from build123d import *

# Parameters (mm, degrees)
F0_R     = 3.3
F1_DEPTH = 5
F2_W     = 33
F2_H     = 6.5
F2_W_2   = 28
F3_DEPTH = 2


# Not quite as in the source:
# - a feature names something its author has since deleted; it is built from what else it names


with BuildPart() as f1:
    # F0 (on Front) → F1 (new body)
    with BuildSketch(Plane.XZ):
        Polygon((0, 17), (0, 0), (80, 0), (80, 17), (80, 23), (80, 25), (0, 25), (0, 23), align=None)
        with Locations((7, 7)):
            Circle(F0_R, mode=Mode.SUBTRACT)
        with Locations((73, 7)):
            Circle(F0_R, mode=Mode.SUBTRACT)
    extrude(amount=F1_DEPTH)

    # F2 (on face) → F3 (cut)
    with BuildSketch(Plane.XZ.offset(5)):
        with Locations((22.3, 20.25)):
            Rectangle(F2_W, F2_H)
        with Locations((60.3, 20.25)):
            Rectangle(F2_W_2, F2_H)
    extrude(amount=-F3_DEPTH, mode=Mode.SUBTRACT)


solid = f1.part
Verification items for the finished model (mm, model axes). A direction names the side the tool comes from. Coordinates: 2 decimals unless noted, no trailing zeros. Write each loop counter-clockwise with the first axis right and the second up, starting at its lowest first coordinate (ties: lowest second). Pieces come first, ordered by that corner, then holes. Notation, with made-up numbers: (-16.75, 43.5) - (13.25, 43.5) arc R30 ccw to (13.25, 67.5) - close; hole circle Ø8 at (-8, 40). An arc over 180 degrees is marked (long way). Answer as a JSON object with one key per item and string values.
(1) Tool access check on faces 5 (the flat face through (5.8, -4, 20)), 6 (the cylindrical face through (69.7, -2.5, 7.1)). Record the directions out of +Z, -Z, +X, -X, +Y, -Y that give a thin tool (end or side, any length) a straight path to the whole face; none if there is none.
Report:
{"face 5": "-Y", "face 6": "+Y, -Y"}
(2) Cross-section at C-C on y = -4.05. Record the cut outline in (x, z), plus the area to 3 significant figures.
Report:
{"outline": "(0, 0) - (80, 0) - (80, 25) - (0, 25) - close; hole circle Ø6.6 at (7, 7); hole (5.8, 17) - (38.8, 17) - (38.8, 23.5) - (5.8, 23.5) - close; hole (46.3, 17) - (74.3, 17) - (74.3, 23.5) - (46.3, 23.5) - close; hole circle Ø6.6 at (73, 7)", "area": "1,540 mm^2"}
(3) Cross-section at A-A on z = 7. Record the cut outline in (x, y).
Report:
{"outline": "(0, -5) - (3.7, -5) - (3.7, 0) - (0, 0) - close; (10.3, -5) - (69.7, -5) - (69.7, 0) - (10.3, 0) - close; (76.3, -5) - (80, -5) - (80, 0) - (76.3, 0) - close"}
(4) Mould release check, pull along Z, two halves, no side actions. Record for faces 1 (the flat face through (39, -5, 13)), 2 (the flat face through (60, -4, 17)), 3 (the flat face through (22, -4, 17)), 4 (the flat face through (41, -2, 25)): pulls with the +Z half, pulls with the -Z half, needs draft (parallel to the pull), parting line crosses it, or undercut.
Report:
{"face 1": "needs draft", "face 2": "undercut", "face 3": "undercut", "face 4": "pulls with the +Z half"}
(5) Gauge pin test, flat ends, axial feed: pin 1 Ø3 at (x, z) = (28, 21) entering from -Y; pin 2 Ø6 at (x, z) = (73, 7) entering from +Y. Record the tip position at first contact, or that the pin passes through.
Report:
{"pin 1": "y = -3", "pin 2": "through"}
(6) Cross-section at B-B on x = 73. Record the cut outline in (y, z), plus the area to 3 significant figures.
Report:
{"outline": "(-5, 0) - (0, 0) - (0, 3.7) - (-5, 3.7) - close; (-5, 10.3) - (0, 10.3) - (0, 25) - (-5, 25) - (-5, 23.5) - (-3, 23.5) - (-3, 17) - (-5, 17) - close", "area": "79.0 mm^2"}
(7) Thickness scan on line 1 along Z through (x, y) = (7, -3.55); line 2 along X through (y, z) = (-3.55, 9.5); line 3 along Z through (x, y) = (73, -1.85). Record the ranges inside material, lowest first.
Report:
{"line 1": "0 to 3.7, 10.3 to 17, 23.5 to 25", "line 2": "0 to 4.85, 9.15 to 70.85, 75.15 to 80", "line 3": "0 to 3.7, 10.3 to 25"}
(8) Cross-section at D-D on x = 21.5. Record the cut outline in (y, z), plus the area to 3 significant figures.
Report:
{"outline": "(-5, 0) - (0, 0) - (0, 25) - (-5, 25) - (-5, 23.5) - (-3, 23.5) - (-3, 17) - (-5, 17) - close", "area": "112 mm^2"}
